Here's how the part is built. I have some questions about the finished solid (model axes, mm). Coordinates: 2 decimals unless noted, no trailing zeros. Write each loop counter-clockwise with the first axis right and the second up, starting at its lowest first coordinate (ties: lowest second). Pieces come first, ordered by that corner, then holes.
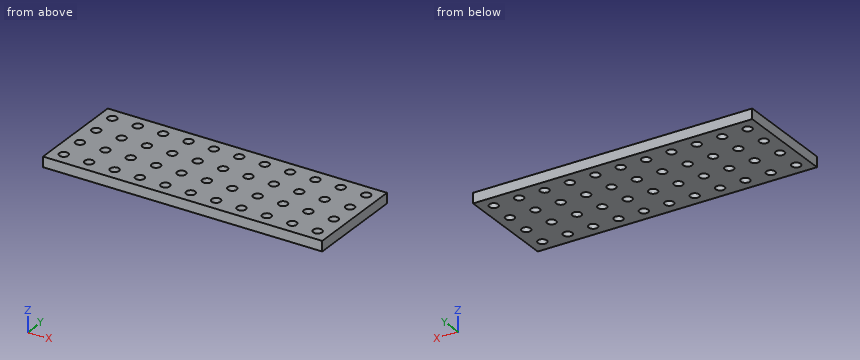
from build123d import *

# Parameters (mm, degrees)
ESQUISSE1_W        = 110
ESQUISSE1_H        = 40
ESQUISSE1_R        = 1.75
BOSS_EXTRU_1_DEPTH = 4


with BuildPart() as part:
    # Esquisse1 → Boss.-Extru.1 (new body)
    with BuildSketch(Plane.XY):
        with Locations((55, -20)):
            Rectangle(ESQUISSE1_W, ESQUISSE1_H)
        with Locations((5, -5)):
            Circle(ESQUISSE1_R, mode=Mode.SUBTRACT)
        with Locations((15, -5)):
            Circle(ESQUISSE1_R, mode=Mode.SUBTRACT)
        with Locations((25, -5)):
            Circle(ESQUISSE1_R, mode=Mode.SUBTRACT)
        with Locations((35, -5)):
            Circle(ESQUISSE1_R, mode=Mode.SUBTRACT)
        with Locations((45, -5)):
            Circle(ESQUISSE1_R, mode=Mode.SUBTRACT)
        with Locations((55, -5)):
            Circle(ESQUISSE1_R, mode=Mode.SUBTRACT)
        with Locations((65, -5)):
            Circle(ESQUISSE1_R, mode=Mode.SUBTRACT)
        with Locations((75, -5)):
            Circle(ESQUISSE1_R, mode=Mode.SUBTRACT)
        with Locations((85, -5)):
            Circle(ESQUISSE1_R, mode=Mode.SUBTRACT)
        with Locations((95, -5)):
            Circle(ESQUISSE1_R, mode=Mode.SUBTRACT)
        with Locations((105, -5)):
            Circle(ESQUISSE1_R, mode=Mode.SUBTRACT)
        with Locations((15, -15)):
            Circle(ESQUISSE1_R, mode=Mode.SUBTRACT)
        with Locations((25, -15)):
            Circle(ESQUISSE1_R, mode=Mode.SUBTRACT)
        with Locations((35, -15)):
            Circle(ESQUISSE1_R, mode=Mode.SUBTRACT)
        with Locations((45, -15)):
            Circle(ESQUISSE1_R, mode=Mode.SUBTRACT)
        with Locations((55, -15)):
            Circle(ESQUISSE1_R, mode=Mode.SUBTRACT)
        with Locations((65, -15)):
            Circle(ESQUISSE1_R, mode=Mode.SUBTRACT)
        with Locations((75, -15)):
            Circle(ESQUISSE1_R, mode=Mode.SUBTRACT)
        with Locations((85, -15)):
            Circle(ESQUISSE1_R, mode=Mode.SUBTRACT)
        with Locations((95, -15)):
            Circle(ESQUISSE1_R, mode=Mode.SUBTRACT)
        with Locations((105, -15)):
            Circle(ESQUISSE1_R, mode=Mode.SUBTRACT)
        with Locations((15, -25)):
            Circle(ESQUISSE1_R, mode=Mode.SUBTRACT)
        with Locations((25, -25)):
            Circle(ESQUISSE1_R, mode=Mode.SUBTRACT)
        with Locations((35, -25)):
            Circle(ESQUISSE1_R, mode=Mode.SUBTRACT)
        with Locations((45, -25)):
            Circle(ESQUISSE1_R, mode=Mode.SUBTRACT)
        with Locations((55, -25)):
            Circle(ESQUISSE1_R, mode=Mode.SUBTRACT)
        with Locations((65, -25)):
            Circle(ESQUISSE1_R, mode=Mode.SUBTRACT)
        with Locations((75, -25)):
            Circle(ESQUISSE1_R, mode=Mode.SUBTRACT)
        with Locations((85, -25)):
            Circle(ESQUISSE1_R, mode=Mode.SUBTRACT)
        with Locations((95, -25)):
            Circle(ESQUISSE1_R, mode=Mode.SUBTRACT)
        with Locations((105, -25)):
            Circle(ESQUISSE1_R, mode=Mode.SUBTRACT)
        with Locations((15, -35)):
            Circle(ESQUISSE1_R, mode=Mode.SUBTRACT)
        with Locations((25, -35)):
            Circle(ESQUISSE1_R, mode=Mode.SUBTRACT)
        with Locations((35, -35)):
            Circle(ESQUISSE1_R, mode=Mode.SUBTRACT)
        with Locations((45, -35)):
            Circle(ESQUISSE1_R, mode=Mode.SUBTRACT)
        with Locations((55, -35)):
            Circle(ESQUISSE1_R, mode=Mode.SUBTRACT)
        with Locations((65, -35)):
            Circle(ESQUISSE1_R, mode=Mode.SUBTRACT)
        with Locations((75, -35)):
            Circle(ESQUISSE1_R, mode=Mode.SUBTRACT)
        with Locations((85, -35)):
            Circle(ESQUISSE1_R, mode=Mode.SUBTRACT)
        with Locations((95, -35)):
            Circle(ESQUISSE1_R, mode=Mode.SUBTRACT)
        with Locations((105, -35)):
            Circle(ESQUISSE1_R, mode=Mode.SUBTRACT)
        with Locations((5, -15)):
            Circle(ESQUISSE1_R, mode=Mode.SUBTRACT)
        with Locations((5, -25)):
            Circle(ESQUISSE1_R, mode=Mode.SUBTRACT)
        with Locations((5, -35)):
            Circle(ESQUISSE1_R, mode=Mode.SUBTRACT)
    extrude(amount=BOSS_EXTRU_1_DEPTH)


solid = part.part
1. If I drill on line 1 (Y direction, x = 35, z = 1.3); line 2 (Y direction, x = 96.5, z = 0.3), over which ranges is the centre line in solid material (lowest first)?
2. I want a section at A-A (x = 55). List the corners of the cut face in (y, z) for me.
3. I want a section at B-B (y = -25). State how many separate pieces and enclosed holes the cut face has, then the cut area to 3 significant figures.
Response values:
1. line 1: y = -40 to -36.75, -33.25 to -26.75, -23.25 to -16.75, -13.25 to -6.75, -3.25 to 0
1. line 2: y = -40 to -35.9, -34.1 to -25.9, -24.1 to -15.9, -14.1 to -5.9, -4.1 to 0
2. outline: (-40, 0) - (-36.75, 0) - (-36.75, 4) - (-40, 4) - close; (-33.25, 0) - (-26.75, 0) - (-26.75, 4) - (-33.25, 4) - close; (-23.25, 0) - (-16.75, 0) - (-16.75, 4) - (-23.25, 4) - close; (-13.25, 0) - (-6.75, 0) - (-6.75, 4) - (-13.25, 4) - close; (-3.25, 0) - (0, 0) - (0, 4) - (-3.25, 4) - close
3. separate pieces: 12
3. enclosed holes: 0
3. area: 286 mm2
